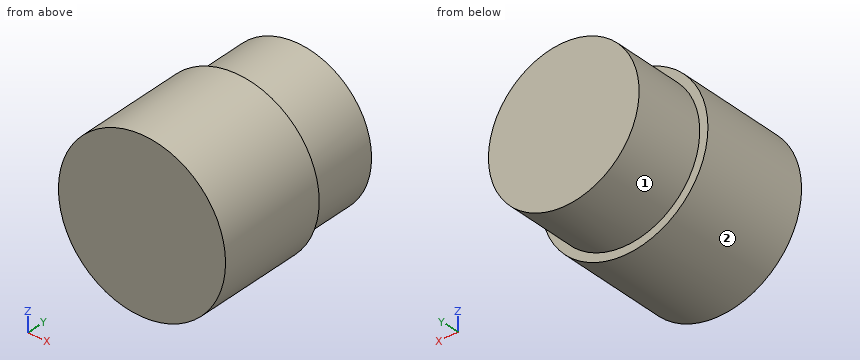
from build123d import *

# Parameters (mm, degrees)
SKETCH067_R             = 2.25
PAD046_DEPTH            = 2.2
SKETCH068_R             = 2.495
PAD047_DEPTH            = 3.4
POCKET019_DEPTH         = 4.4
POLARPATTERN_COUNT      = 80
BODY011_PLACEMENT_ANGLE = 90


with BuildPart() as part:
    # Sketch067 → Pad046 (new body)
    with BuildSketch(Plane.XY):
        Circle(SKETCH067_R)
    extrude(amount=PAD046_DEPTH)

    # Sketch068 (on Face3 of Pad046) → Pad047 (join)
    with BuildSketch(Plane.XY.offset(2.2)):
        Circle(SKETCH068_R)
    extrude(amount=PAD047_DEPTH)

    # Sketch069 (on Face3 of Pad047) → Pocket019 (cut)
    with BuildSketch(Plane.XY.offset(5.6)):
        Polygon((3.3, 0.172946), (3, 0), (3.3, -0.172946), align=None)
    pocket019 = extrude(amount=-POCKET019_DEPTH, mode=Mode.SUBTRACT)

    # PolarPattern: Pocket019 ×80 about axis
    polarpattern_axis = Axis((0, 0, 5.6), (0, 0, 1))
    for i in range(1, POLARPATTERN_COUNT):
        add(pocket019.rotate(polarpattern_axis, i * 360 / POLARPATTERN_COUNT), mode=Mode.SUBTRACT)


with BuildPart() as part_1:
    # Body011 placement: moved
    add(part.part.moved(Location((0.4, 26.3, 17.4))).rotate(Axis((0.4, 26.3, 17.4), (1, 0, 0)), BODY011_PLACEMENT_ANGLE))


solid = part_1.part
Verification items for the finished model (mm, model axes). Face numbers are marked on the shaded views. A direction names the side the tool comes from. Give positions to 0.01 mm unless a question says otherwise; leave off trailing zeros. Write each loop counter-clockwise with the first axis right and the second up, starting at its lowest first coordinate (ties: lowest second). Pieces come first, ordered by that corner, then holes.
(1) Access from +Z, -Z, +X, -X, +Y, -Y to the whole of each face (thin tool, end or side, straight path). Record for the marked faces 1 and 2.
(2) Gauge pin test, flat end, axial feed: pin 1 (1.5 mm diameter, centred on x = 0, y = 25.5, fed in from +Z). Record the tip position at first contact, or that the pin passes through.
(3) Cross-section at D-D (y = 22.1). Enter the section's corners in (x, z) (3 decimals).
(4) Cross-section at C-C (y = 25.5). Enter the section's corners in (x, z), plus the area to 3 significant figures.
(5) Cross-section at B-B (z = 17.4). Enter the section's corners in (x, y) (3 decimals), plus the area to 3 significant figures.
(6) Cross-section at A-A (x = 0.4). Enter the section's corners in (y, z) (3 decimals).
(7) Material ranges on line 1 (Z direction, x = -0.95, y = 24.65); line 2 (X direction, y = 25.6, z = 19.1); line 3 (X direction, y = 26.05, z = 17.3), recorded low to high.
Worked out:
1. face 1: +Y
1. face 2: +Y, -Y
2. pin 1: stops at z = 19.65
3. outline: circle Ø4.99 at (0.4, 17.4)
4. outline: circle Ø4.5 at (0.4, 17.4)
4. area: 15.9 mm2
5. outline: (-2.095, 20.7) - (2.895, 20.7) - (2.895, 24.1) - (2.65, 24.1) - (2.65, 26.3) - (-1.85, 26.3) - (-1.85, 24.1) - (-2.095, 24.1) - close
5. area: 26.9 mm2
6. outline: (20.7, 14.905) - (24.1, 14.905) - (24.1, 15.15) - (26.3, 15.15) - (26.3, 19.65) - (24.1, 19.65) - (24.1, 19.895) - (20.7, 19.895) - close
7. line 1: z = 15.6 to 19.2
7. line 2: x = -1.07 to 1.87
7. line 3: x = -1.85 to 2.65
